```python
from build123d import *

# Parameters (mm, degrees)
BOSS_EXTRUDE1_DEPTH = 4.7625
CAVITY1_START       = -30
CAVITY1_OUTLINE_W   = 4.7625
CAVITY1_OUTLINE_H   = 4.7625
CAVITY1_DEPTH       = 20
CAVITY1_START_2     = 10
CAVITY1_2_OUTLINE_W = 4.7625
CAVITY1_2_OUTLINE_H = 4.7625
CAVITY1_2_DEPTH     = 20


# Read off the part's stored shape, not the designer's step: Cavity1
with BuildPart() as part:
    # Sketch1 → Boss-Extrude1 (new body)
    with BuildSketch(Plane.XY):
        Polygon((50, 40), (50, 60), (45.2375, 60), (45.2375, 80), (50, 80), (50, 100), (-50, 100), (-50, 80), (-45.2375, 80), (-45.2375, 60), (-50, 60), (-50, 40), (-45.2375, 40), (-45.2375, 20), (-50, 20), (-50, 0), (-30, 0), (-30, 4.7625), (-10, 4.7625), (-10, 0), (10, 0), (10, 4.7625), (30, 4.7625), (30, 0), (50, 0), (50, 20), (45.2375, 20), (45.2375, 40), align=None)
    extrude(amount=BOSS_EXTRUDE1_DEPTH)

    # Cavity1 outline → Cavity1 (cut)
    with BuildSketch(Plane.YZ.offset(CAVITY1_START)):
        with Locations((97.61875, 2.38125)):
            Rectangle(CAVITY1_OUTLINE_W, CAVITY1_OUTLINE_H)
    extrude(amount=CAVITY1_DEPTH, mode=Mode.SUBTRACT)

    # Cavity1 2 outline → Cavity1 2 (cut)
    with BuildSketch(Plane.YZ.offset(CAVITY1_START_2)):
        with Locations((97.61875, 2.38125)):
            Rectangle(CAVITY1_2_OUTLINE_W, CAVITY1_2_OUTLINE_H)
    extrude(amount=CAVITY1_2_DEPTH, mode=Mode.SUBTRACT)


solid = part.part
```
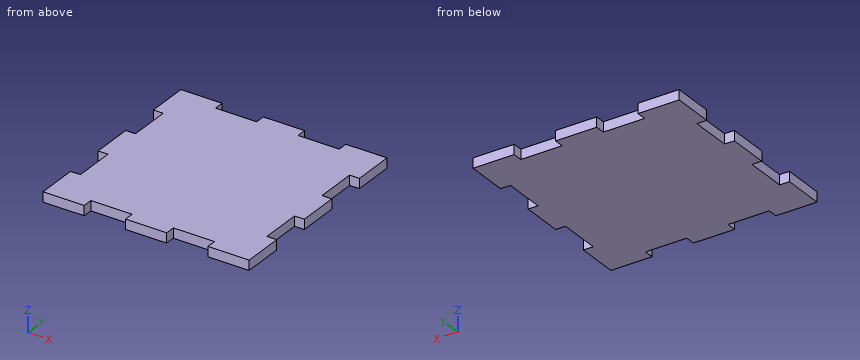
Input: part model. Units: mm. Frame: model coordinates. Give positions to 0.01 mm unless a question says otherwise; leave off trailing zeros. Loops run counter-clockwise (first coordinate to the right, second up) from the corner with the lowest first, then second, coordinate; pieces in that order, holes last.
1) Section query B-B on x = -17.5. Return the cut outline in (y, z), and give its area (3 significant figures).
A:
outline: (4.76, 0) - (95.24, 0) - (95.24, 4.76) - (4.76, 4.76) - close
area: 431 mm2
2) Line query: L1, parallel to Y at x = 11.5, z = 1.75; L2, parallel to X at y = 31, z = 2.05. Output: solid intervals per line, ascending.
A:
L1: y = 4.76 to 95.24
L2: x = -45.24 to 45.24
3) Section query A-A on y = 34.5. Return the cut outline in (x, z).
A:
outline: (-45.24, 0) - (45.24, 0) - (45.24, 4.76) - (-45.24, 4.76) - close
4) Contact query for flat-ended pins moving along their axis: pin 1 (1.4 mm diameter, centred on x = -22.5, z = 2, fed in from -Y); pin 2 (8 mm diameter, centred on x = 33.5, y = 14, fed in from -Z); pin 3 (2.5 mm diameter, centred on x = 21.5, z = 1.5, fed in from +Y). Output: stop coordinate, or through.
A:
pin 1: stops at y = 4.76
pin 2: stops at z = 0
pin 3: stops at y = 95.24
